```python
from build123d import *

# Parameters (mm, degrees)
F0_W     = 4.5
F0_H     = 2.2
F0_R     = 1.1
F1_DEPTH = 0.6
F2_W     = 4.5
F2_H     = 2.2
F3_DEPTH = 1.6
F4_R     = 1.09999
F5_R     = 0.5
F6_DEPTH = 10


# Not quite as in the source:
# - a fillet or chamfer is up to 0.001 mm smaller than in the source, because OpenCascade refuses the exact size


with BuildPart() as f1:
    # F0 (on Top) → F1 (new body)
    with BuildSketch(Plane.XY):
        with Locations((9.75, 2.6)):
            Rectangle(F0_W, F0_H)
        with BuildLine():
            Line((7.0565025569, 1.5), (7.5, 1.5))
            Line((7.5, 1.5), (7.5, 3.7))
            Line((7.5, 3.7), (7.0565025569, 3.7))
            ThreePointArc((7.0565025569, 3.7), (6.7766250144, 3.7151076306), (6.5, 3.7602549529))
            ThreePointArc((6.5, 3.7602549529), (6.2418088438, 3.8309365837), (5.9922537502, 3.9277912239))
            Line((5.9922537502, 3.9277912239), (3.6642488067, 4.9722087761))
            ThreePointArc((3.6642488067, 4.9722087761), (3.1441769851, 5.1424144841), (2.6, 5.2))
            ThreePointArc((2.6, 5.2), (0.7615223689, 4.4384776311), (0, 2.6))
            ThreePointArc((0, 2.6), (0.7615223689, 0.7615223689), (2.6, 0))
            ThreePointArc((2.6, 0), (3.1441769851, 0.0575855159), (3.6642488067, 0.2277912239))
            Line((3.6642488067, 0.2277912239), (5.9922537502, 1.2722087761))
            ThreePointArc((5.9922537502, 1.2722087761), (6.2418088438, 1.3690634163), (6.5, 1.4397450471))
            ThreePointArc((6.5, 1.4397450471), (6.7766250144, 1.4848923694), (7.0565025569, 1.5))
        make_face()
        with Locations((2.6, 2.6)):
            Circle(F0_R, mode=Mode.SUBTRACT)
    extrude(amount=F1_DEPTH)

    # F2 (on face) → F3 (join)
    with BuildSketch(Plane.XY.offset(0.6)):
        with Locations((9.75, 2.6)):
            Rectangle(F2_W, F2_H)
    extrude(amount=F3_DEPTH)

    # F4 (radius 1.1 in the source; OpenCascade refuses exactly that, so slightly less here)
    f4_edges = [f1.edges().sort_by_distance(p)[0] for p in [
        (9.75, 1.5, 2.2),
        (9.75, 3.7, 2.2),
    ]]
    fillet(f4_edges, radius=F4_R)

    # F5 (on face) → F6 (cut)
    with BuildSketch(Plane.YZ.offset(12)):
        with Locations((2.6, 1.1)):
            Circle(F5_R)
    extrude(amount=-F6_DEPTH, mode=Mode.SUBTRACT)


solid = f1.part
```
Here's how the part is built. I have some questions about the finished solid (model axes, mm). A direction names the side the tool comes from. Give positions to 0.01 mm unless a question says otherwise; leave off trailing zeros. Loops run counter-clockwise (first coordinate to the right, second up) from the corner with the lowest first, then second, coordinate; pieces in that order, holes last. Notation, with made-up numbers: M -10,13 L 21,13 A28 cw 21,31 Z; hole C -16,59 d2. An arc over 180 degrees is marked long. Return JSON: item names as keys, results as strings.
Item 1: Imagine slicing it at D-D on z = 1.3. List the corners of the cut face in (x, y) for me.
A:
{"outline": "M 7.5,1.52 L 12,1.52 L 12,2.14 L 7.5,2.14 Z; M 7.5,3.06 L 12,3.06 L 12,3.68 L 7.5,3.68 Z"}
Item 2: Imagine slicing it at B-B on x = 2.75. List the corners of the cut face in (y, z) for me.
A:
{"outline": "M 0,0 L 1.51,0 L 1.51,0.6 L 0,0.6 Z; M 3.69,0 L 5.2,0 L 5.2,0.6 L 3.69,0.6 Z"}
Item 3: I'm going to push flat-ended pins straight in: pin 1 Ø3 at (x, y) = (2.6, 2.6) entering from +Z; pin 2 Ø0.9 at (x, z) = (10, 0.5) entering from +Y; pin 3 Ø0.6 at (x, z) = (9.5, 1) entering from -Y. Where does each tip first touch, or does it pass through?
A:
{"pin 1": "stops at z = 0.6", "pin 2": "stops at y = 3.7", "pin 3": "stops at y = 1.5"}
Item 4: Thinking about a two-plate mould opening in Z: for faces 4 (the flat face through (7.5, 2.3, 1.7)), 5 (the flat face through (5, 3, 0)), 6 (the flat face through (4, 3, 0.6)), 7 (the cylindrical face through (9.8, 2.9, 1.5)), which applies, released by +Z, released by -Z, zero draft, split by the parting line, or undercut?
A:
{"face 4": "zero draft", "face 5": "released by -Z", "face 6": "released by +Z", "face 7": "undercut"}
Item 5: Please list where these lines run through material, in increasing order: line 1 (Z direction, x = 9.55, y = 2.6); line 2 (Y direction, x = 10.8, z = 1.1); line 3 (Y direction, x = 2.6, z = 0.1).
A:
{"line 1": "z = 0 to 0.6, 1.6 to 2.2", "line 2": "y = 1.5 to 2.1, 3.1 to 3.7", "line 3": "y = 0 to 1.5, 3.7 to 5.2"}
Item 6: Imagine slicing it at A-A on z = 0.25. List the corners of the cut face in (x, y) for me, then the cut area to 3 significant figures.
A:
{"outline": "M 3.66,0.23 L 5.99,1.27 A2.6 cw 7.06,1.5 L 12,1.5 L 12,3.7 L 7.06,3.7 A2.6 cw 5.99,3.93 L 3.66,4.97 A2.6 ccw long Z; hole C 2.6,2.6 d2.2", "area": "34.2 mm^2"}
Item 7: On a 3-axis mill with a long thin cutter (end or side, diameter ignored), from which of +Z, -Z, +X, -X, +Y, -Y can I reach the whole of each face in a straight line? I mean faces 1 (the flat face through (9.5, 3.7, 0.5)), 2 (the flat face through (9.5, 1.5, 0.5)), 3 (the cylindrical face through (2.362, 1.526, 0.296)). Say none if no direction works.
A:
{"face 1": "+Z, -Z, +X, +Y", "face 2": "+Z, -Z, +X, -Y", "face 3": "+Z, -Z"}
